CAD build for the part. Positions are in the model's coordinates, mm. Face numbers are marked on the shaded views. A direction names the side the tool comes from. Coordinates: 2 decimals unless noted, no trailing zeros. Write each loop counter-clockwise with the first axis right and the second up, starting at its lowest first coordinate (ties: lowest second). Pieces come first, ordered by that corner, then holes.
Autodesk Inventor part; units mm, degrees
ref_plane "YZ Plane" through (0, 0, 0) normal (1, 0, 0) x (0, 1, 0)
ref_plane "XZ Plane" through (0, 0, 0) normal (0, 1, 0) x (-1, 0, 0)
ref_plane "XY Plane" through (0, 0, 0) normal (0, 0, 1) x (1, 0, 0)
sketch "Sketch1" plane through (0, 0, 0) normal (0, 1, 0) x (-1, 0, 0)
  line L0 (23.5, 27) -> (-23.5, 27)
  line L1 (-23.5, -27) -> (23.5, -27)
  line L2 (23.5, -27) -> (23.5, 27)
  line L3 (21.5, 25) -> (-21.5, 25)
  line L4 (-21.5, -25) -> (21.5, -25)
  line L5 (21.5, -25) -> (21.5, 25)
  line L6 (-21.5, -25) -> (-21.5, -19)
  line L7 (-21.5, -19) -> (-23.5, -19)
  line L8 (-21.5, 25) -> (-21.5, 19)
  line L9 (-21.5, 19) -> (-23.5, 19)
  line L10 (-23.5, 27) -> (-23.5, 19)
  line L11 (-23.5, -19) -> (-23.5, -27)
  line L12 (-21.5, 25) -> (-21.5, 19)
  line L13 (-21.5, -19) -> (-21.5, -25)
  dimension "d2" = 47
  dimension "d3" = 54
  dimension "d4" = 43
  dimension "d5" = 50
  dimension "d6" = 6
  dimension "d7" = 6
extrude "Extrusion1" add sketch "Sketch1" along normal blind 4.5
sketch "Sketch2" plane through (0, 4.5, 0) normal (0, 1, 0) x (1, 0, 0)
  line L0 (23.5, -27) -> (-23.5, -27)
  line L1 (23.5, 27) -> (-23.5, 27)
  line L2 (-23.5, -27) -> (-23.5, 27)
  line L3 (-23.5, 27) -> (23.5, 27)
  line L4 (23.5, 19) -> (23.5, 27)
  line L5 (23.5, 27) -> (23.5, 19)
  line L6 (23.5, 19) -> (21.5, 19)
  line L7 (21.5, 25) -> (21.5, 19)
  line L8 (21.5, 19) -> (21.5, 25)
  line L9 (21.5, 25) -> (-21.5, 25)
  line L10 (-21.5, -25) -> (-21.5, 25)
  line L11 (-21.5, 25) -> (-21.5, -25)
  line L12 (-21.5, -25) -> (21.5, -25)
  line L13 (21.5, -25) -> (21.5, -19)
  line L14 (21.5, -19) -> (23.5, -19)
  line L15 (23.5, -27) -> (23.5, -19)
  line L16 (23.5, -19) -> (23.5, -27)
  line L17 (21.5, -25) -> (-21.5, -25)
  line L18 (-21.5, -25) -> (-19.5, -25)
  circle A0 centre (-19.5, -23) radius 1.5
  circle A1 centre (-19.5, -23) radius 2
  line L19 (-21.5, 25) -> (-19.5, 25)
  line L20 (-21.5, 25) -> (21.5, 25)
  circle A2 centre (-19.5, 23) radius 1.5
  circle A3 centre (-19.5, 23) radius 2
  line L21 (21.5, 25) -> (19.5, 25)
  circle A4 centre (19.5, 23) radius 1.5
  circle A5 centre (19.5, 23) radius 2
  line L22 (21.5, -25) -> (19.5, -25)
  circle A6 centre (19.5, -23) radius 1.5
  circle A7 centre (19.5, -23) radius 2
  point P0 (0, 0)
  dimension "d13" = 2
extrude "Extrusion2" add sketch "Sketch2" along normal blind 11 contours L0 L2 L1 L4 L6 L7 L9 L10 L12 L13 L14 L15 | A7 | A1 | A5 | A3
sketch "Sketch3" plane through (0, 15.5, 0) normal (0, 1, 0) x (1, 0, 0)
  point P0 (0, 0)
sketch "Sketch4" plane through (0, 15.5, 0) normal (0, 1, 0) x (1, 0, 0)
  circle A0 centre (-19.5, -23) radius 1.5
  circle A1 centre (-19.5, -23) radius 1.5
  circle A2 centre (-19.5, 23) radius 1.5
  circle A3 centre (-19.5, 23) radius 1.5
  arc A4 (19.5, 25) -> (21.5, 23) centre (19.5, 23) ccw
  circle A5 centre (19.5, 23) radius 1.5
  circle A6 centre (19.5, -23) radius 1.5
  circle A7 centre (19.5, -23) radius 1.5
  line L0 (23.5, 27) -> (-23.5, 27)
  line L1 (23.5, -27) -> (-23.5, -27)
  line L2 (-23.5, -27) -> (-23.5, 27)
  line L3 (-23.5, 27) -> (23.5, 27)
  line L4 (23.5, 19) -> (23.5, 27)
  line L5 (23.5, 19) -> (13.5, 19)
  line L6 (23.5, -27) -> (23.5, -19)
  line L7 (23.5, -19) -> (13.5, -19)
  line L8 (13.5, -19) -> (13.5, 19)
  line L9 (23.5, 27) -> (23.5, 19)
  line L10 (23.5, -19) -> (23.5, -27)
  line L11 (-23.5, 27) -> (-23.5, -27)
  line L12 (-21.5, -25) -> (-21.5, 25)
  line L13 (-19.5, 25) -> (19.5, 25)
  line L14 (-15.5, 23) -> (2, 23)
  line L15 (2, 23) -> (2, 19.5)
  line L16 (2, 19.5) -> (-15.5, 19.5)
  line L17 (-15.5, 19.5) -> (-15.5, 23)
  point P0 (0, 0)
  dimension "d24" = 10
  dimension "d25" = 10
  dimension "d31" = 17.5
  dimension "d32" = 3.5
extrude "Extrusion3" add sketch "Sketch4" along normal blind 2
sketch "Sketch5" plane through (-23.5, 0, -27) normal (-1, 0, 0) x (0, 0, 1)
  point P0 (27, 0)
sketch "Sketch6" plane through (-23.5, 0, -27) normal (-1, 0, 0) x (0, 0, 1)
  point P0 (27, 0)
sketch "Sketch7" plane through (0, 17.5, 0) normal (0, 1, 0) x (1, 0, 0)
  circle A0 centre (-3.8686, -11.2916) radius 2.7
  arc A1 (0.181, -6.4655) -> (-8.6946, -7.242) centre (-3.8686, -11.2916) ccw
  arc A2 (1.9165, -4.3972) -> (-10.763, -5.5065) centre (-3.8686, -11.2916) ccw
  arc A3 (4.2306, -1.6394) -> (-13.5207, -3.1924) centre (-3.8686, -11.2916) ccw
  arc A4 (5.9661, 0.4289) -> (-15.589, -1.4569) centre (-3.8686, -11.2916) ccw
  arc A5 (8.2801, 3.1867) -> (-18.3468, 0.8571) centre (-3.8686, -11.2916) ccw
  arc A6 (10.0162, 5.2557) -> (-20.2878, 2.7444) centre (-3.8686, -11.2916) ccw
  line L0 (-20.2878, 2.7444) -> (-20.4151, 2.5927)
  line L1 (-20.4151, 2.5927) -> (-20.2871, 2.4853)
  line L2 (-18.3468, 0.8571) -> (-20.2871, 2.4853)
  line L3 (-13.5207, -3.1924) -> (-15.589, -1.4569)
  line L4 (-8.6946, -7.242) -> (-10.763, -5.5065)
  line L5 (0.181, -6.4655) -> (1.9165, -4.3972)
  line L6 (4.2306, -1.6394) -> (5.9661, 0.4289)
  line L7 (8.2801, 3.1867) -> (10.0162, 5.2557)
  dimension "d58" = 5.4
extrude "Extrusion4" cut sketch "Sketch7" against normal through all
properties part number "Box1_Top"
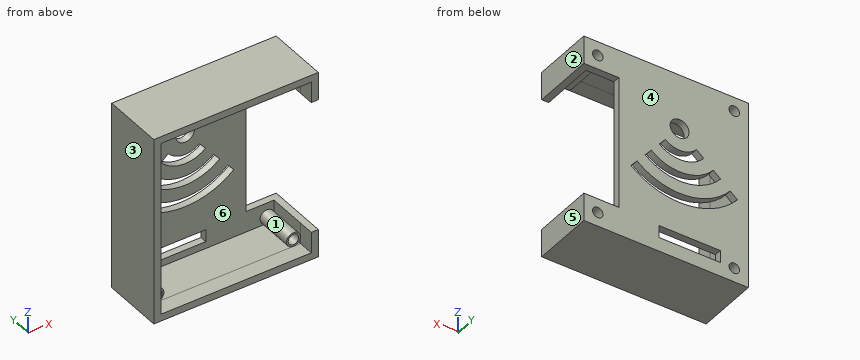
Item 1: Saw through at D-D, the plane y = 3.5. Write the cut outline in (x, z), and give its area (3 significant figures).
Item 2: Which spindle directions (+Z, -Z, +X, -X, +Y, -Y) get a long thin tool onto all of the face, cutting with end or side? Do the marked faces 5 and 6. Say none if no direction does.
Item 3: Two-plate mould, pull along X, no slides. Class the marked faces 1, 2, 3 and 4: +X half, -X half, draft (parallel to the pull), parting line (faces both ways), or undercut.
Item 4: Wall check: line 1 along Z through (x, y) = (-10, 7); line 2 along X through (y, z) = (1.5, 21.5); line 3 along Z through (x, y) = (18.5, 11). Give the ranges that are in metal, low to high.
Item 5: Saw through at C-C, the plane z = -14. Write the cut outline in (x, y), and give its area (3 significant figures).
Item 6: Saw through at B-B, the plane x = -8. Write the cut outline in (y, z).
Item 7: Flat gauge pins, fed straight in: pin 1 Ø12 at (x, z) = (-6.5, -11) entering from -Y; pin 2 Ø9 at (y, z) = (10, -0.5) entering from +X; pin 3 Ø1 at (x, z) = (-20.5, -24) entering from -Y. Where does each tip first touch, or does it go through?
Working result:
1. outline: (-23.5, -27) - (23.5, -27) - (23.5, -19) - (21.5, -19) - (21.5, -25) - (-21.5, -25) - (-21.5, 25) - (21.5, 25) - (21.5, 19) - (23.5, 19) - (23.5, 27) - (-23.5, 27) - close
1. area: 312 mm2
2. face 5: +Z, -Z, +X, +Y, -Y
2. face 6: -Y
3. face 1: undercut
3. face 2: +X half
3. face 3: -X half
3. face 4: draft
4. line 1: z = -27 to -25, 25 to 27
4. line 2: x = -23.5 to -21.5, 21.5 to 23.5
4. line 3: z = -27 to -25, -24.73 to -24.12, -21.88 to -21.27, 21.27 to 21.88, 24.12 to 24.73, 25 to 27
5. outline: (-23.5, 0) - (-21.5, 0) - (-21.5, 15.5) - (13.5, 15.5) - (13.5, 17.5) - (-23.5, 17.5) - close
5. area: 105 mm2
6. outline: (0, -27) - (17.5, -27) - (17.5, -23) - (15.5, -23) - (15.5, -25) - (0, -25) - close; (0, 25) - (15.5, 25) - (15.5, 6.54) - (17.5, 6.54) - (17.5, 27) - (0, 27) - close; (15.5, -19.5) - (17.5, -19.5) - (17.5, -9.91) - (15.5, -9.91) - close; (15.5, -7.15) - (17.5, -7.15) - (17.5, -3.44) - (15.5, -3.44) - close; (15.5, -0.61) - (17.5, -0.61) - (17.5, 3.3) - (15.5, 3.3) - close
7. pin 1: stops at y = 15.5
7. pin 2: stops at x = -21.5
7. pin 3: stops at y = 4.5
